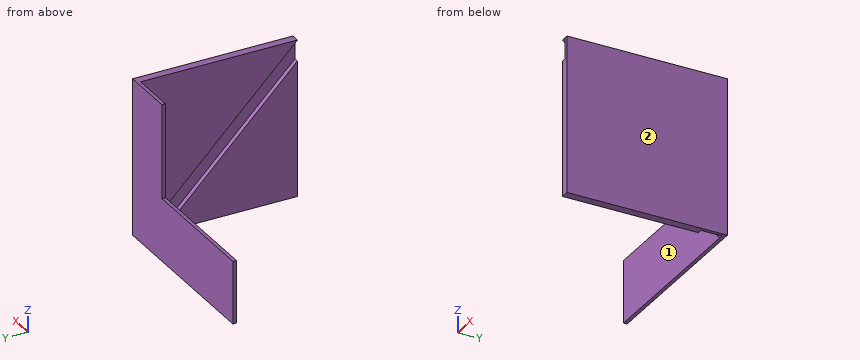
Autodesk Inventor part; units mm, degrees
ref_plane "YZ Plane" through (0, 0, 0) normal (1, 0, 0) x (0, 1, 0)
ref_plane "XZ Plane" through (0, 0, 0) normal (0, 1, 0) x (-1, 0, 0)
ref_plane "XY Plane" through (0, 0, 0) normal (0, 0, 1) x (1, 0, 0)
sketch "Sketch1" plane through (0, 0, 0) normal (0, 1, 0) x (-1, 0, 0)
  line L0 (110, -80) -> (-110, -80)
  line L1 (-110, -80) -> (-110, 80)
  line L2 (-110, 80) -> (110, 80)
  line L3 (110, 80) -> (110, -80)
  line L4 (320.2117, -53.5522) -> (168.036, -53.5522) construction
  line L5 (168.036, -53.5522) -> (168.036, 90.1689) construction
  line L6 (168.036, 90.1689) -> (320.2117, 90.1689) construction
  line L7 (320.2117, 90.1689) -> (320.2117, -53.5522) construction
  line L8 (124.3, -89.75) -> (-124.3, -89.75) construction
  line L9 (-124.3, -89.75) -> (-124.3, 89.75) construction
  line L10 (-124.3, 89.75) -> (124.3, 89.75) construction
  line L11 (124.3, 89.75) -> (124.3, -89.75) construction
  line L12 (124.3, -89.75) -> (-124.3, 89.75) construction
  line L13 (-124.3, -89.75) -> (124.3, 89.75) construction
  line L14 (-152.4, -107.95) -> (152.4, -107.95)
  line L15 (152.4, -107.95) -> (152.4, 107.95)
  line L16 (152.4, 107.95) -> (-152.4, 107.95)
  line L17 (-152.4, 107.95) -> (-152.4, -107.95)
  line L18 (-152.4, -107.95) -> (152.4, 107.95) construction
  line L19 (152.4, -107.95) -> (-152.4, 107.95) construction
  line L20 (177.8, 133.35) -> (177.8, -133.35)
  line L21 (177.8, -133.35) -> (-177.8, -133.35)
  line L22 (-177.8, -133.35) -> (-177.8, 133.35)
  line L23 (-177.8, 133.35) -> (177.8, 133.35)
  point P0 (0, 0)
  dimension "d11" = 220
  dimension "d12" = 160
  dimension "d15" = 248.6
  dimension "d16" = 179.5
  dimension "d18" = 304.8
  dimension "d19" = 215.9
  dimension "d22" = 25.4
extrude "Top" add sketch "Sketch1" along normal blind 25.4 contours L17 L16 L15 L14 | L20 L21 L22 L23
sketch "Sketch3" plane through (177.8, 0, 133.35) normal (1, 0, 0) x (0, 0, -1)
  line L0 (0, 0) -> (0, 25.4)
  line L1 (266.7, 0) -> (266.7, 25.4)
  line L2 (0, 0) -> (266.7, 0)
  line L3 (266.7, 0) -> (266.7, -266.7)
  line L4 (266.7, -266.7) -> (0, -266.7)
  line L5 (0, -266.7) -> (0, 0)
  point P0 (133.35, 0)
  dimension "d25" = 266.7
extrude "Right" add sketch "Sketch3" against normal blind 50.8
sketch "Sketch4" plane through (-177.8, 0, -133.35) normal (-1, 0, 0) x (0, 0, 1)
  line L0 (0, 0) -> (0, 25.4)
  line L1 (266.7, -266.7) -> (266.7, 0)
  line L2 (0, 0) -> (266.7, 0)
  line L3 (266.7, 0) -> (266.7, -266.7)
  line L4 (266.7, -266.7) -> (0, -266.7)
  line L5 (0, -266.7) -> (0, 0)
  point P0 (133.35, 0)
  dimension "d28" = 266.7
extrude "Left" add sketch "Sketch4" against normal blind 50.8
sketch "Sketch5" plane through (0, 0, 0) normal (1, 0, 0) x (0, 1, 0)
  line L0 (-266.7, -133.35) -> (25.4, -133.35)
  line L1 (-266.7, 133.35) -> (-266.7, -133.35)
  line L2 (0, -133.35) -> (-266.7, 133.35)
  line L3 (-266.7, 133.35) -> (-275.6803, 124.3697)
  line L4 (-275.6803, 124.3697) -> (-8.9803, -142.3303)
  line L5 (-8.9803, -142.3303) -> (0, -133.35)
  point P0 (0, 0)
  dimension "d31" = 12.7
extrude "Plexiglass Cut" cut sketch "Sketch5" along normal mid plane 304.8 contours L4 L1 L2 L0 | L0 L5 L4 | L4 L3 L1
sketch "Sketch6" plane through (-177.8, -266.7, -133.35) normal (0, -1, 0) x (1, 0, 0)
  line L0 (0, 0) -> (0, 266.7)
  line L1 (355.6, 0) -> (0, 0)
  line L2 (0, 266.7) -> (355.6, 266.7)
  line L3 (355.6, 266.7) -> (355.6, 0)
  line L4 (355.6, 0) -> (0, 0)
  line L5 (0, 0) -> (0, 266.7)
  point P0 (177.8, 133.35)
extrude "Bottom" add sketch "Sketch6" along normal blind 25.4
sketch "Sketch9" plane through (0, 25.4, 0) normal (0, 1, 0) x (1, 0, 0)
  line L0 (177.8, -133.35) -> (127, -133.35)
  line L1 (177.8, 133.35) -> (-177.8, 133.35)
  line L2 (177.8, -133.35) -> (-177.8, -133.35)
  line L3 (-177.8, -133.35) -> (-177.8, 133.35)
  line L4 (-177.8, 133.35) -> (177.8, 133.35)
  line L5 (177.8, 133.35) -> (177.8, -133.35)
  point P0 (0, 0)
extrude "Top Flattening" cut sketch "Sketch9" against normal blind 22.4
sketch "Sketch10" plane through (0, 3, 0) normal (0, 1, 0) x (1, 0, 0)
  line L0 (-177.8, -133.35) -> (-177.8, 133.35)
  line L1 (-155.4106, 133.35) -> (-177.8, 133.35)
  line L2 (-177.8, 133.35) -> (-177.8, -133.35)
  line L3 (-177.8, -133.35) -> (-155.4106, -133.35)
  line L4 (-155.4106, -133.35) -> (-155.4106, 133.35)
  line L5 (177.8, 133.35) -> (177.8, -133.35)
  line L6 (177.8, -133.35) -> (155.4106, -133.35)
  line L7 (155.4106, -133.35) -> (155.4106, 133.35)
  line L8 (155.4106, 133.35) -> (177.8, 133.35)
  line L9 (152.4, -115.3895) -> (152.4, 133.35)
  point P0 (0, 0)
  point P1 (-177.8, 0)
  dimension "d48" = 22.3894
  dimension "d49" = 22.3894
extrude "Outer Side Flattening" cut sketch "Sketch10" against normal through all
sketch "Sketch11" plane through (-177.8, -292.1, -133.35) normal (0, -1, 0) x (1, 0, 0)
  line L0 (22.3894, 0) -> (333.2106, 0)
  line L1 (333.2106, 0) -> (22.3894, 0)
  line L2 (22.3894, 0) -> (22.3894, 266.7)
  line L3 (22.3894, 266.7) -> (333.2106, 266.7)
  line L4 (333.2106, 266.7) -> (333.2106, 0)
  point P0 (177.8, 133.35)
extrude "Bottom Flattening" cut sketch "Sketch11" against normal blind 22.4
sketch "Sketch12" plane through (155.4106, 3, -133.35) normal (0, 0, -1) x (-1, 0, 0)
  line L0 (155.4106, -3) -> (155.4106, -269.7) construction
  line L1 (7.0106, -269.7) -> (7.0106, -3)
  line L2 (7.0106, -3) -> (303.8106, -3)
  line L3 (303.8106, -3) -> (303.8106, -269.7)
  line L4 (303.8106, -269.7) -> (7.0106, -269.7)
  line L5 (7.0106, -269.7) -> (303.8106, -3) construction
  line L6 (7.0106, -3) -> (303.8106, -269.7) construction
  point P0 (155.4106, -136.35)
  point P1 (155.4106, -3)
  dimension "d54" = 296.8
extrude "Inner Flattening" cut sketch "Sketch12" against normal through all
sketch "Sketch13" plane through (-155.4106, 3, 133.35) normal (0, 0, 1) x (1, 0, 0)
  line L0 (310.8211, -272.7) -> (310.8211, 0)
  line L1 (0, -272.7) -> (310.8211, -272.7)
  line L2 (310.8211, -136.35) -> (0, -136.35)
  line L3 (0, -136.35) -> (0, -272.7)
  line L4 (0, -272.7) -> (310.8211, -272.7)
  line L5 (310.8211, -272.7) -> (310.8211, -136.35)
  point P0 (155.4106, -3)
extrude "Bottom Cut" cut sketch "Sketch13" against normal through all
sketch "Sketch14" plane through (0, 3, 0) normal (0, 1, 0) x (1, 0, 0)
  line L0 (-155.4106, 133.35) -> (155.4106, 133.35)
  line L1 (0, 0) -> (155.4106, 0)
  line L2 (155.4106, 0) -> (155.4106, 133.35)
  line L3 (155.4106, 133.35) -> (0, 133.35)
  line L4 (0, 133.35) -> (0, 0)
  line L5 (155.4106, -133.35) -> (-155.4106, -133.35)
  line L6 (155.4106, 133.35) -> (-155.4106, 133.35)
  line L7 (-155.4106, 133.35) -> (-155.4106, -133.35)
  line L8 (-155.4106, -133.35) -> (155.4106, -133.35)
  line L9 (155.4106, -133.35) -> (155.4106, 133.35)
extrude "Quarter Cut" cut sketch "Sketch14" against normal through all contours L0 L4 L1 L9 L5 L7
properties part number "Apple iPad 2022 Hologram"
Input: part model. Units: mm. Frame: model coordinates. Face numbers are marked on the shaded views. A direction names the side the tool comes from. Give positions to 0.01 mm unless a question says otherwise; leave off trailing zeros. Order: outer loops, then holes, each group sorted by start corner. A loop starts at its lowest first (then second) coordinate and runs counter-clockwise, first axis right, second up. Notation, with made-up numbers: M 58.5,8 L 83.5,8 A19 ccw 83.5,38 Z; hole C 19.25,79.5 d7. An arc over 180 degrees is marked long. One line per question, with ' | ' between items. Start each with the question number.
1. Section query D-D (z = -41.5). Return the cut outline in (x, y), and give its area (3 significant figures).
2. Material intervals for probe 1 along Y at (x, z) = (55, -107); probe 2 along X at (y, z) = (-24, -88.5); probe 3 along X at (y, z) = (-71.5, -74), sorted ascending. Write a range as [from, to].
3. Section query C-C (x = 97.5). Return the cut outline in (y, z), and give its area (3 significant figures).
4. Section query B-B (y = -116.5). Return the cut outline in (x, z), and give its area (3 significant figures).
5. First-contact query: pin 1 Ø2.5 at (x, y) = (74, 1.5) entering from +Z; pin 2 Ø2.5 at (y, z) = (1.5, -34) entering from -X; pin 3 Ø1.5 at (y, z) = (-39, -107.5) entering from -X. Flat tips, straight axial feed; report the tip coordinate or a pass-through.
6. Section query A-A (z = -13). Return the cut outline in (x, y), and give its area (3 significant figures).
7. Access query for the marked faces 1 and 2. Directions: +Z, -Z, +X, -X, +Y, -Y. A direction counts if a zero-diameter tool reaches every point of the face in a straight line with its end or side. Return the directions, or none.
Here are the results:
1) outline: M 110,0 L 148.4,0 L 148.4,-91.85 L 152.4,-91.85 L 152.4,-109.81 L 148.4,-109.81 L 148.4,-133.35 L 155.41,-133.35 L 155.41,3 L 110,3 Z | area: 999 mm²
2) probe 1: [0, 3] | probe 2: [148.4, 155.41] | probe 3: [152.4, 155.41]
3) outline: M 0,-133.35 L 3,-133.35 L 3,-80 L 0,-80 Z | area: 160 mm²
4) outline: M 148.4,-133.35 L 155.41,-133.35 L 155.41,0 L 148.4,0 L 148.4,-16.85 L 152.4,-16.85 L 152.4,-34.81 L 148.4,-34.81 Z | area: 863 mm²
5) pin 1: z = -80 | pin 2: x = 110 | pin 3: x = 152.4
6) outline: M 110,0 L 148.4,0 L 148.4,-120.35 L 152.4,-120.35 L 152.4,-133.35 L 155.41,-133.35 L 155.41,3 L 110,3 Z | area: 1,020 mm²
7) face 1: +Z, -Z, -X, -Y | face 2: +Z, -Z, +X, +Y, -Y
